```python
from build123d import *

# Parameters (mm, degrees)
F1_DEPTH      = 25.4
F1_DEPTH_BACK = 25.4
F2_SIZE       = 7.62
F3_R          = 7.62
F4_R          = 7.62


with BuildPart() as f1:
    # F0 (on Front) → F1 (new body, two sides)
    with BuildSketch(Plane.XZ) as f1_sk:
        Polygon((-20.073232, 22.875223), (-6.280771, 43.673378), (-17.396271, 66.017077), (-42.304232, 67.562621), (-56.096693, 46.764467), (-44.981193, 24.420768), align=None)
    extrude(amount=F1_DEPTH)
    extrude(f1_sk.sketch, amount=-F1_DEPTH_BACK)

    # F2
    f2_edges = [f1.edges().sort_by_distance(p)[0] for p in [
        (-29.850251, -25.4, 66.789849),
        (-11.838521, -25.4, 54.845227),
        (-13.177002, -25.4, 33.2743),
        (-49.200462, -25.4, 57.163544),
        (-50.538943, -25.4, 35.592617),
        (-32.527213, -25.4, 23.647995),
        (-13.177002, 25.4, 33.2743),
        (-11.838521, 25.4, 54.845227),
        (-29.850251, 25.4, 66.789849),
        (-49.200462, 25.4, 57.163544),
        (-50.538943, 25.4, 35.592617),
        (-32.527213, 25.4, 23.647995),
    ]]
    chamfer(f2_edges, length=F2_SIZE)

    # F3
    f3_edges = [f1.edges().sort_by_distance(p)[0] for p in [
        (-30.322166, -25.4, 59.184476),
        (-18.660925, -25.4, 51.451231),
        (-42.849974, -25.4, 52.952167),
        (-19.52749, -25.4, 37.485677),
        (-43.716539, -25.4, 38.986613),
        (-32.055298, -25.4, 31.253368),
    ]]
    fillet(f3_edges, radius=F3_R)

    # F4
    f4_edges = [f1.edges().sort_by_distance(p)[0] for p in [
        (-19.52749, 25.4, 37.485677),
        (-32.055298, 25.4, 31.253368),
        (-18.660925, 25.4, 51.451231),
        (-43.716539, 25.4, 38.986613),
        (-30.322166, 25.4, 59.184476),
        (-42.849974, 25.4, 52.952167),
    ]]
    fillet(f4_edges, radius=F4_R)


solid = f1.part
```
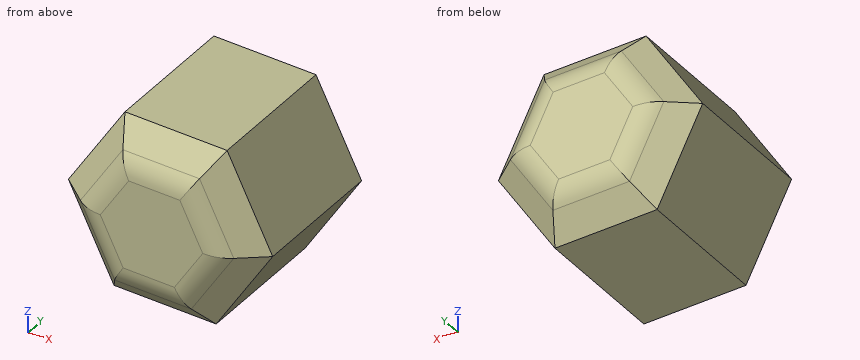
Build history of the part. All positions in model axes, mm. Round coordinates to 2 decimals unless told otherwise and drop trailing zeros. Write each loop counter-clockwise with the first axis right and the second up, starting at its lowest first coordinate (ties: lowest second). Pieces come first, ordered by that corner, then holes.
1) Drill centre lines: probe 1 along Z at (x, y) = (-24.5, -14.5); probe 2 along X at (y, z) = (2.5, 45); probe 3 along X at (y, z) = (-4, 54). Where is each one in solid material? Low to high.
2) Pin check, flat tips, straight feed: pin 1 (4 mm diameter, centred on y = 14.5, z = 36, fed in from -X); pin 2 (1.5 mm diameter, centred on x = -50, z = 52, fed in from -Y); pin 3 (5 mm diameter, centred on y = 0.5, z = 34, fed in from +X). Stop position of each tip, or through.
3) Band-saw the part on B-B, the plane y = -20. List the corners of the cut face in (x, z) (1 decimal), and give its area (3 significant figures).
4) Band-saw the part on A-A, the plane y = 16.5. List the corners of the cut face in (x, z), and give its area (3 significant figures).
Ans:
1. probe 1: z = 23.15 to 66.46
1. probe 2: x = -55.22 to -6.94
1. probe 3: x = -51.3 to -11.42
2. pin 1: stops at x = -51.74
2. pin 2: stops at y = -20.72
2. pin 3: stops at x = -11.04
3. outline: (-53.5, 46.6) - (-43.6, 26.6) - (-21.2, 25.2) - (-8.8, 43.8) - (-18.8, 63.9) - (-41.2, 65.3) - close
3. area: 1,300 mm2
4. outline: (-56.1, 46.76) - (-44.98, 24.42) - (-20.07, 22.88) - (-6.28, 43.67) - (-17.4, 66.02) - (-42.3, 67.56) - close
4. area: 1,620 mm2
